```python
from build123d import *

# Parameters (mm, degrees)
SKETCH1_W           = 82
SKETCH1_H           = 25
BOSS_EXTRUDE1_DEPTH = 14.2
CUT_EXTRUDE3_DEPTH  = 14.2
BOSS_EXTRUDE2_DEPTH = 1
BOSS_EXTRUDE3_START = -13.2
BOSS_EXTRUDE3_DEPTH = 1
CUT_EXTRUDE4_START  = -4.5
CUT_EXTRUDE4_DEPTH  = 3.25
CUT_EXTRUDE5_DEPTH  = 4.5
CUT_EXTRUDE6_DEPTH  = 14.2
SKETCH8_R           = 1.625
CUT_EXTRUDE7_DEPTH  = 5


with BuildPart() as part:
    # Sketch1 → Boss-Extrude1 (new body)
    with BuildSketch(Plane.XY):
        with Locations((0, 12.5)):
            Rectangle(SKETCH1_W, SKETCH1_H)
    extrude(amount=BOSS_EXTRUDE1_DEPTH)

    # Sketch2 → Cut-Extrude3 (cut)
    with BuildSketch(Plane(origin=(0, 0, 0), x_dir=(-1, 0, 0), z_dir=(0, 0, -1))):
        with BuildLine():
            Line((-31, 0), (-19, 0))
            ThreePointArc((-19, 0), (-25, 6), (-31, 0))
        make_face()
        with BuildLine():
            Line((19, 0), (31, 0))
            ThreePointArc((31, 0), (25, 6), (19, 0))
        make_face()
    extrude(amount=-CUT_EXTRUDE3_DEPTH, mode=Mode.SUBTRACT)

    # Sketch4 → Boss-Extrude2 (add)
    with BuildSketch(Plane(origin=(0, 0, 0), x_dir=(-1, 0, 0), z_dir=(0, 0, -1))):
        with BuildLine():
            Line((-30.75, 0), (-31, 0))
            ThreePointArc((-31, 0), (-25, 6), (-19, 0))
            Line((-19, 0), (-19.25, 0))
            ThreePointArc((-19.25, 0), (-25, 5.75), (-30.75, 0))
        make_face()
        with BuildLine():
            Line((19, 0), (19.25, 0))
            ThreePointArc((19.25, 0), (25, 5.75), (30.75, 0))
            Line((30.75, 0), (31, 0))
            ThreePointArc((31, 0), (25, 6), (19, 0))
        make_face()
    extrude(amount=-BOSS_EXTRUDE2_DEPTH)

    # Sketch4<2> → Boss-Extrude3 (add)
    with BuildSketch(Plane(origin=(0, 0, 0), x_dir=(-1, 0, 0), z_dir=(0, 0, -1)).offset(BOSS_EXTRUDE3_START)):
        with BuildLine():
            Line((-30.75, 0), (-31, 0))
            ThreePointArc((-31, 0), (-25, 6), (-19, 0))
            Line((-19, 0), (-19.25, 0))
            ThreePointArc((-19.25, 0), (-25, 5.75), (-30.75, 0))
        make_face()
        with BuildLine():
            Line((19, 0), (19.25, 0))
            ThreePointArc((19.25, 0), (25, 5.75), (30.75, 0))
            Line((30.75, 0), (31, 0))
            ThreePointArc((31, 0), (25, 6), (19, 0))
        make_face()
    extrude(amount=-BOSS_EXTRUDE3_DEPTH)

    # Sketch5 → Cut-Extrude4 (cut)
    with BuildSketch(Plane(origin=(0, 0, 0), x_dir=(-1, 0, 0), z_dir=(0, 0, -1)).offset(CUT_EXTRUDE4_START)):
        with BuildLine():
            Line((-6.5, 0), (6.5, 0))
            ThreePointArc((6.5, 0), (0, 6.5), (-6.5, 0))
        make_face()
    extrude(amount=-CUT_EXTRUDE4_DEPTH, mode=Mode.SUBTRACT)

    # Sketch6 → Cut-Extrude5 (cut)
    with BuildSketch(Plane(origin=(0, 0, 0), x_dir=(-1, 0, 0), z_dir=(0, 0, -1))):
        with BuildLine():
            Line((-2.625, 0), (2.625, 0))
            ThreePointArc((2.625, 0), (0, 2.625), (-2.625, 0))
        make_face()
    extrude(amount=-CUT_EXTRUDE5_DEPTH, mode=Mode.SUBTRACT)

    # Sketch7 → Cut-Extrude6 (cut)
    with BuildSketch(Plane(origin=(0, 0, 0), x_dir=(-1, 0, 0), z_dir=(0, 0, -1))):
        with BuildLine():
            Line((-41, 5), (-33.5, 5))
            ThreePointArc((-33.5, 5), (-29.896033736, 8.560306867), (-25, 9.861541462))
            Line((-25, 9.861541462), (25, 9.861541462))
            ThreePointArc((25, 9.861541462), (29.896033736, 8.560306867), (33.5, 5))
            Line((33.5, 5), (41, 5))
            Line((41, 5), (41, 25))
            Line((41, 25), (-41, 25))
            Line((-41, 25), (-41, 5))
        make_face()
    extrude(amount=-CUT_EXTRUDE6_DEPTH, mode=Mode.SUBTRACT)

    # Sketch8 → Cut-Extrude7 (cut)
    with BuildSketch(Plane(origin=(0, 5, 0), x_dir=(1, 0, 0), z_dir=(0, 1, 0))):
        with Locations(Location((37.25, -3.75, 0), (0, 0, 270))):
            Circle(SKETCH8_R)
        with Locations(Location((37.25, -10.45, 0), (0, 0, 270))):
            Circle(SKETCH8_R)
        with Locations(Location((-37.25, -3.75, 0), (0, 0, 270))):
            Circle(SKETCH8_R)
        with Locations(Location((-37.25, -10.45, 0), (0, 0, 270))):
            Circle(SKETCH8_R)
    extrude(amount=-CUT_EXTRUDE7_DEPTH, mode=Mode.SUBTRACT)


solid = part.part
```
Source: CAD feature listing. Evaluate the final solid. Frame: model axes, mm. A direction names the side the tool comes from. Give positions to 0.01 mm unless a question says otherwise; leave off trailing zeros. Loops run counter-clockwise (first coordinate to the right, second up) from the corner with the lowest first, then second, coordinate; pieces in that order, holes last. Notation, with made-up numbers: M -12.75,35 L 43.25,35 A3 ccw 43.25,39 Z; hole C 25,41.25 d1. An arc over 180 degrees is marked long. Put each result on its own line as item: value.
Q1. Mould query, pull axis Z, two halves, no side actions, for faces 4 (the flat face through (0, 0, 9)), 5 (the flat face through (-1, 5, 14.2)), 6 (the flat face through (0, 3, 4.5)), 7 (the cylindrical face through (35.81, 2.54, 11.2)). Classes: released by +Z, released by -Z, zero draft, split by the parting line, or undercut.
Response values:
face 4: zero draft
face 5: released by +Z
face 6: undercut
face 7: undercut
Q2. Line query: probe 1 along X at (y, z) = (5.5, 8.5); probe 2 along X at (y, z) = (3.5, 13.25); probe 3 along X at (y, z) = (3.6, 10.45) (3 decimals). Output: solid intervals per line, ascending. Write a range as [from, to].
Response values:
probe 1: x = [-33.19, -27.4], [-22.6, 22.6], [27.4, 33.19]
probe 2: x = [-41, -29.56], [-20.44, 20.44], [29.56, 41]
probe 3: x = [-41, -38.875], [-35.625, -29.8], [-20.2, 20.2], [29.8, 35.625], [38.875, 41]
Q3. Section B-B (x = 37.25). Return the cut outline in (y, z) (3 decimals).
Response values:
outline: M 0,0 L 5,0 L 5,2.125 L 0,2.125 Z; M 0,5.375 L 5,5.375 L 5,8.825 L 0,8.825 Z; M 0,12.075 L 5,12.075 L 5,14.2 L 0,14.2 Z
Q4. Pin query (flat end, axial travel): P1, Ø2, axis at y = 8.5, z = 10.5, coming from the +X side; P2, Ø3.5, axis at x = 37.25, z = 3.75, coming from the +Y side. Return the tip coordinate at first contact, or that it passes through.
Response values:
P1: stops at x = 31.4
P2: stops at y = 5
Q5. Section A-A (z = 10.45). Return the cut outline in (x, y) (3 decimals), and give its area (3 significant figures).
Response values:
outline: M -41,0 L -38.875,0 L -38.875,5 L -41,5 Z; M -35.625,0 L -31,0 A6 cw -19,0 L 19,0 A6 cw 31,0 L 35.625,0 L 35.625,5 L 33.5,5 A9.862 ccw 25,9.862 L -25,9.862 A9.862 ccw -33.5,5 L -35.625,5 Z; M 38.875,0 L 41,0 L 41,5 L 38.875,5 Z
area: 566 mm²
Q6. Section C-C (x = 0). Return the cut outline in (y, z) (3 decimals).
Response values:
outline: M 0,7.75 L 6.5,7.75 L 6.5,4.5 L 2.625,4.5 L 2.625,0 L 9.862,0 L 9.862,14.2 L 0,14.2 Z
Q7. Section D-D (z = 3.5). Return the cut outline in (x, y) (3 decimals).
Response values:
outline: M -41,0 L -38.856,0 L -38.856,5 L -41,5 Z; M -35.644,0 L -31,0 A6 cw -19,0 L -2.625,0 A2.625 cw 2.625,0 L 19,0 A6 cw 31,0 L 35.644,0 L 35.644,5 L 33.5,5 A9.862 ccw 25,9.862 L -25,9.862 A9.862 ccw -33.5,5 L -35.644,5 Z; M 38.856,0 L 41,0 L 41,5 L 38.856,5 Z
Q8. Reachability of faces 1 (the flat face through (-37, 5, 7)), 2 (the flat face through (0, 3, 7.75)), 3 (the flat face through (37, 5, 7)) from +Z, -Z, +X, -X, +Y, -Y: full face, straight path, thin tool, end or side. Return the list, or none.
Response values:
face 1: +Z, -Z, -X, +Y
face 2: -Y
face 3: +Z, -Z, +X, +Y
